Part model, mm, in its own coordinate system. A direction names the side the tool comes from. Coordinates: 2 decimals unless noted, no trailing zeros. Loops run counter-clockwise (first coordinate to the right, second up) from the corner with the lowest first, then second, coordinate; pieces in that order, holes last. Notation, with made-up numbers: (76, -21) -> (81, -21) arc R11 ccw to (81, -2) -> close; hole circle Ø7 at (-28, -30.75). An arc over 180 degrees is marked (long way). One line per question, with ' | ' between items. Start each with the question number.
1) Cut at B-B (z = 25.5). List the corners of the cut face in (x, y).
2) Cut at D-D (x = 142). List the corners of the cut face in (y, z).
3) Drop flat-ended pins along their axis: pin 1 (10.5 mm diameter, centred on y = 113, z = 25, fed in from +X); pin 2 (1.2 mm diameter, centred on y = 171.5, z = -3, fed in from -X); pin 3 (4 mm diameter, centred on x = 77, z = 26.5, fed in from -Y); pin 4 (3 mm diameter, centred on y = 61.5, z = -1.5, fed in from -X). Give the stop position or say it passes through.
4) 3-axis set-ups, long thin cutter, end or side, ignore diameter. For faces 5 (the face through (76, 175, 21)), 6 (the face through (87, 220, -1)), 7 (the face through (30.703, 41.014, -2.028)), 8 (the face through (75.972, 201.345, 26.409)), 9 (the face through (78, 203, 25)): which of +Z, -Z, +X, -X, +Y, -Y reach the whole face in a straight line?
5) Cut at A-A (x = 90). List the corners of the cut face in (y, z), plus the area to 3 significant figures.
6) Probe L1, parallel to Y at x = 102, z = -0.95; L2, parallel to Y at x = 277, z = -2; L3, parallel to Y at x = 77, z = -1. List the from-to ranges inside material, lowest first. Write a range as from..to.
7) Cut at C-C (y = 141). List the corners of the cut face in (x, z).
8) Two-plate mould, pull along X, no slides. Class faces 1 (the face through (208.986, 40.703, -2.028)), 2 (the face through (308, 104.76, -1.97)), 3 (the face through (230, 0, -1)), 4 (the face through (76.406, 197.815, -1.719)): released by +X, released by -X, zero draft, split by the parting line, or undercut.
from build123d import *

# Parameters (mm, degrees)
SKETCH_1_W                  = 190
SKETCH_1_H                  = 55
SM_BASE_FLANGE_1_DEPTH      = 4
SKETCH_6_R                  = 32.5
SKETCH_6_R_2                = 2.5
CUT_EXTRUDE_1_DEPTH         = 10
SKETCH_7_R                  = 5
CUT_EXTRUDE_2_DEPTH         = 10
FILLET_1_R                  = 20
FILLET_2_R                  = 20
SM_EDGE_FLANGE_1_DEPTH      = 45
SM_EDGE_FLANGE_1_BEND_DEPTH = 170
CUT_EXTRUDE_4_REACH         = 525.684
SKETCH_15_R                 = 6.5


# Sheet-metal steps are written as plain solids
with BuildPart() as part:
    # Sketch 1 → 基体-法兰1 (new body)
    with BuildSketch(Plane.XY):
        with BuildLine():
            Line((0, 0), (0, 170))
            Line((0, 170), (82, 170))
            Line((82, 170), (82, 220))
            Line((82, 220), (121.626028344, 220))
            ThreePointArc((121.626028344, 220), (190, 165), (258.373971656, 220))
            Line((258.373971656, 220), (306.965193707, 220))
            ThreePointArc((306.965193707, 220), (343.344749394, 91.076951546), (465, 35))
            Line((465, 35), (465, 0))
            Line((465, 0), (0, 0))
        make_face()
        with Locations((120, 62.5)):
            Rectangle(SKETCH_1_W, SKETCH_1_H, mode=Mode.SUBTRACT)
    extrude(amount=-SM_BASE_FLANGE_1_DEPTH)

    # 草图6 → 切除-拉伸1 (cut)
    with BuildSketch(Plane.XY):
        with Locations((277, 95)):
            Circle(SKETCH_6_R)
        with Locations((277, 133)):
            Circle(SKETCH_6_R_2)
        with Locations((309.908965344, 76)):
            Circle(SKETCH_6_R_2)
        with Locations((244.091034656, 76)):
            Circle(SKETCH_6_R_2)
    extrude(amount=-CUT_EXTRUDE_1_DEPTH, mode=Mode.SUBTRACT)

    # 草图7 → 切除-拉伸2 (cut)
    with BuildSketch(Plane.XY):
        with Locations((20, 95)):
            Circle(SKETCH_7_R)
        with Locations((102, 193.5)):
            Circle(SKETCH_7_R)
        with Locations((277, 193.5)):
            Circle(SKETCH_7_R)
    extrude(amount=-CUT_EXTRUDE_2_DEPTH, mode=Mode.SUBTRACT)

    # 圆角1
    fillet_1_edges = [part.edges().sort_by_distance(p)[0] for p in [
        (25, 35, -2),
        (25, 90, -2),
        (215, 90, -2),
        (215, 35, -2),
    ]]
    fillet(fillet_1_edges, radius=FILLET_1_R)

    # 圆角2
    fillet_2_edges = [part.edges().sort_by_distance(p)[0] for p in [
        (306.965193707, 220, -2),
    ]]
    fillet(fillet_2_edges, radius=FILLET_2_R)

    # 边线-法兰1 section (across the edge) → 边线-法兰1 (add)
    with BuildSketch(Plane(origin=(78, 220, 0), x_dir=(1, 0, 0), z_dir=(0, -1, 0))):
        with BuildLine():
            Line((-4, 4), (-4, 46))
            Line((-4, 46), (0, 46))
            Line((0, 46), (0, 4))
            ThreePointArc((0, 4), (1.171572875, 1.171572875), (4, 0))
            Line((4, 0), (4, -4))
            ThreePointArc((4, -4), (-1.656854249, -1.656854249), (-4, 4))
        make_face()
    extrude(amount=SM_EDGE_FLANGE_1_DEPTH)

    # 边线-法兰1 section 2 (across the edge) → 边线-法兰1 bend (add)
    with BuildSketch(Plane(origin=(-4, 170, 0), x_dir=(1, 0, 0), z_dir=(0, -1, 0))):
        with BuildLine():
            Line((-4, 4), (-4, 46))
            Line((-4, 46), (0, 46))
            Line((0, 46), (0, 4))
            ThreePointArc((0, 4), (1.171572875, 1.171572875), (4, 0))
            Line((4, 0), (4, -4))
            ThreePointArc((4, -4), (-1.656854249, -1.656854249), (-4, 4))
        make_face()
    extrude(amount=SM_EDGE_FLANGE_1_BEND_DEPTH)

    # 草图15 → 切除-拉伸4 (cut, up to next)
    with BuildSketch(Plane.ZY.offset(8), mode=Mode.PRIVATE) as cut_extrude_4_sk1:
        with Locations((25, 113)):
            Circle(SKETCH_15_R)
    cut_extrude_4_tool1 = extrude(cut_extrude_4_sk1.sketch, amount=-CUT_EXTRUDE_4_REACH, mode=Mode.PRIVATE) & part.part
    # 草图15 → 切除-拉伸4 (cut, up to next)
    with BuildSketch(Plane.ZY.offset(8), mode=Mode.PRIVATE) as cut_extrude_4_sk2:
        with Locations(Location((25, 195, 0), (0, 0, 180))):
            Circle(SKETCH_15_R)
    cut_extrude_4_tool2 = extrude(cut_extrude_4_sk2.sketch, amount=-CUT_EXTRUDE_4_REACH, mode=Mode.PRIVATE) & part.part
    add(cut_extrude_4_tool1.solids().sort_by_distance((-8, 113, 25))[0], mode=Mode.SUBTRACT)
    add(cut_extrude_4_tool2.solids().sort_by_distance((-8, 195, 25))[0], mode=Mode.SUBTRACT)


solid = part.part
Reported:
1) outline: (-8, 0) -> (-4, 0) -> (-4, 106.52) -> (-8, 106.52) -> close; (-8, 119.48) -> (-4, 119.48) -> (-4, 170) -> (-8, 170) -> close; (74, 175) -> (78, 175) -> (78, 188.52) -> (74, 188.52) -> close; (74, 201.48) -> (78, 201.48) -> (78, 220) -> (74, 220) -> close
2) outline: (0, -4) -> (35, -4) -> (35, 0) -> (0, 0) -> close; (90, -4) -> (184.05, -4) -> (184.05, 0) -> (90, 0) -> close
3) pin 1: passes through | pin 2: stops at x = 82 | pin 3: stops at y = 175 | pin 4: stops at x = -6.93
4) face 5: +Z, -Z, -X | face 6: +Z, -Z, +X, -X, +Y | face 7: +Z, -Z | face 8: +X, -X | face 9: +Z, +X, +Y, -Y
5) outline: (0, -4) -> (35, -4) -> (35, 0) -> (0, 0) -> close; (90, -4) -> (220, -4) -> (220, 0) -> (90, 0) -> close | area: 660 mm²
6) L1: y = 0..35, 90..188.5, 198.5..220 | L2: y = 0..62.5, 127.5..130.5, 135.5..188.5, 198.5..220 | L3: y = 0..35, 90..170, 175..220
7) outline: (-8, 4) arc R8 ccw to (0, -4) -> (314.39, -4) -> (314.39, 0) -> (0, 0) arc R4 cw to (-4, 4) -> (-4, 46) -> (-8, 46) -> close
8) face 1: undercut | face 2: undercut | face 3: zero draft | face 4: released by -X
